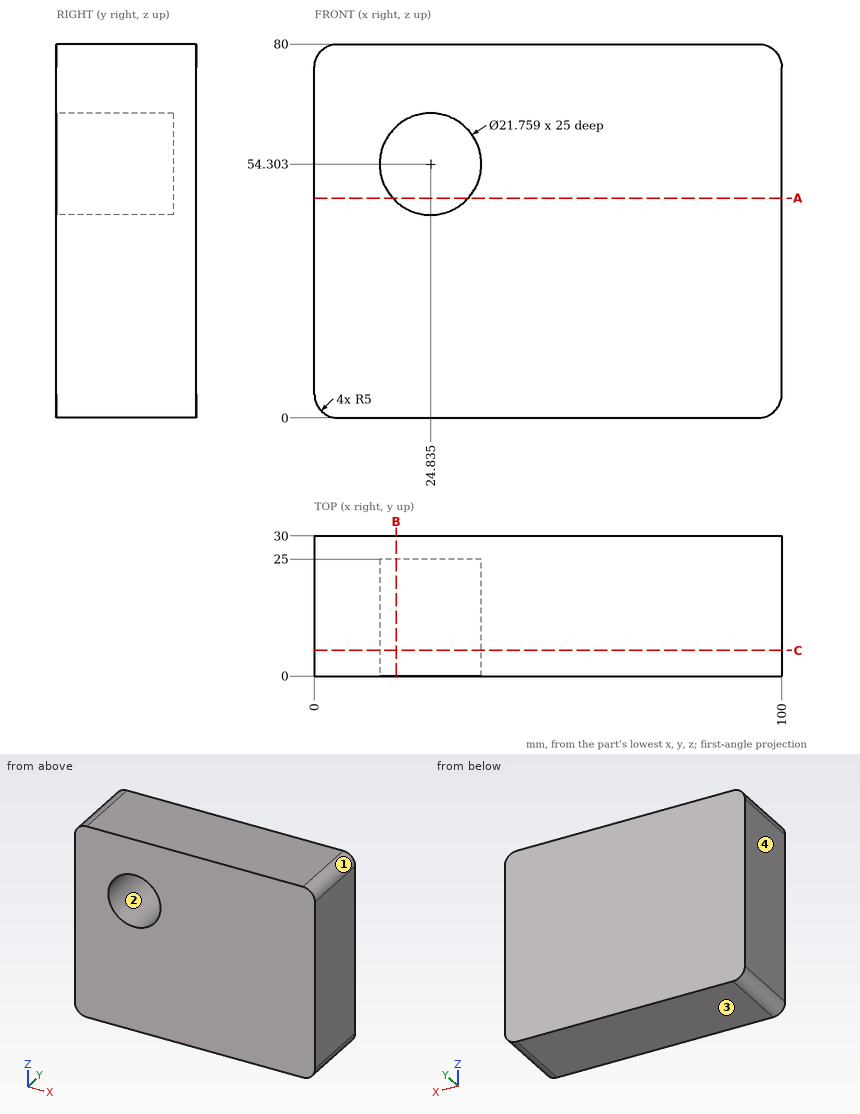
Source: three-view drawing plus pictorial views. Frame: mm from the lowest corner of the part. Give positions to 0.01 mm unless a question says otherwise; leave off trailing zeros. Write each loop counter-clockwise with the first axis right and the second up, starting at its lowest first coordinate (ties: lowest second). Pieces come first, ordered by that corner, then holes.
(1) Cut plane B-B, the plane x = 17.5. Return loops of the section in (y, z), then the cut area to 3 significant figures.
(2) Cut plane C-C, the plane y = 5.5. Return loops of the section in (x, z) (1 decimal).
(3) Ray query, line 1 (X direction, y = 7, z = 63); line 2 (Z direction, x = 16.5, y = 18.25) (1 decimal); line 3 (Z direction, x = 34.5, y = 1.5) (1 decimal). Return the intervals inside material, ascending.
(4) Cut plane A-A, the plane z = 47. Return loops of the section in (x, y), then the cut area to 3 significant figures.
(5) Mould query, pull axis X, two halves, no side actions, for the marked faces 1, 2, 3 and 4. Classes: released by +X, released by -X, zero draft, split by the parting line, or undercut.
Values follow:
1. outline: (0, 0) - (30, 0) - (30, 80) - (0, 80) - (0, 62.34) - (25, 62.34) - (25, 46.27) - (0, 46.27) - close
1. area: 2,000 mm2
2. outline: (0, 5) arc R5 ccw to (5, 0) - (95, 0) arc R5 ccw to (100, 5) - (100, 75) arc R5 ccw to (95, 80) - (5, 80) arc R5 ccw to (0, 75) - close; hole circle Ø21.8 at (24.8, 54.3)
3. line 1: x = 0 to 18.3, 31.37 to 100
3. line 2: z = 0 to 47.3, 61.3 to 80
3. line 3: z = 0 to 49.3, 59.3 to 80
4. outline: (0, 0) - (16.77, 0) - (16.77, 25) - (32.9, 25) - (32.9, 0) - (100, 0) - (100, 30) - (0, 30) - close
4. area: 2,600 mm2
5. face 1: released by +X
5. face 2: undercut
5. face 3: zero draft
5. face 4: released by -X
